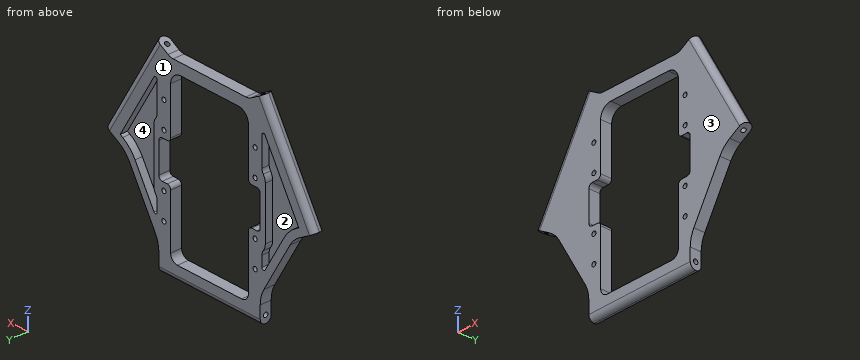
```python
from build123d import *

# Parameters (mm, degrees)
BOSS_EXTRUDE1_DEPTH = 6
SKETCH6_R           = 1.2
CUT_EXTRUDE1_DEPTH  = 104
SKETCH4_R           = 1.2
CUT_EXTRUDE2_DEPTH  = 104
SKETCH2_R           = 1.2
CUT_EXTRUDE3_DEPTH  = 104
FILLET2_R           = 3
SKETCH11_R          = 1.2
BOSS_EXTRUDE3_DEPTH = 32
SKETCH13_R          = 1.2
BOSS_EXTRUDE4_DEPTH = 32
BOSS_EXTRUDE5_START = -32
SKETCH14_R          = 1.2
BOSS_EXTRUDE5_DEPTH = 32
SKETCH16_W          = 46
SKETCH16_H          = 88
CUT_EXTRUDE5_DEPTH  = 10
SKETCH15_R          = 1.2
CUT_EXTRUDE4_DEPTH  = 10
FILLET3_R           = 6
FILLET1_R           = 16
FILLET4_R           = 6
FILLET5_R           = 4
CUT_EXTRUDE6_DEPTH  = 10
FILLET6_R           = 2
SKETCH18_R          = 1.2
CUT_EXTRUDE7_DEPTH  = 10
CUT_EXTRUDE8_DEPTH  = 4


with BuildPart() as part:
    # Sketch1 → Boss-Extrude1 (new body)
    with BuildSketch(Plane(origin=(0, 0, 0), x_dir=(1, 0, 0), z_dir=(0, 1, 0))):
        Polygon((-30, 54), (30, 54), (30, 40.038475773), (49.674337148, 5.961524227), (61.765371804, -1.019237886), (31.765371804, -52.980762114), (23.138438763, -48), (-23.138438763, -48), (-31.765371804, -52.980762114), (-61.765371804, -1.019237886), (-49.674337148, 5.961524227), (-30, 40.038475773), align=None)
    extrude(amount=BOSS_EXTRUDE1_DEPTH)

    # Sketch6 → Cut-Extrude1 (cut)
    with BuildSketch(Plane(origin=(15, 0, -25.980762114), x_dir=(-0.8660254037844389, 0, -0.4999999999999996), z_dir=(0.4999999999999996, 0, -0.8660254037844389))):
        with Locations((-50, 3)):
            Circle(SKETCH6_R)
    extrude(amount=-CUT_EXTRUDE1_DEPTH, mode=Mode.SUBTRACT)

    # Sketch4 → Cut-Extrude2 (cut)
    with BuildSketch(Plane(origin=(-15, 0, -25.980762114), x_dir=(-0.8660254037844386, 0, 0.5), z_dir=(-0.5000000000000001, 0, -0.8660254037844387))):
        with Locations((50, 3)):
            Circle(SKETCH4_R)
    extrude(amount=-CUT_EXTRUDE2_DEPTH, mode=Mode.SUBTRACT)

    # Sketch2 → Cut-Extrude3 (cut)
    with BuildSketch(Plane.ZY.offset(30)):
        with Locations((-50, 3)):
            Circle(SKETCH2_R)
    extrude(amount=-CUT_EXTRUDE3_DEPTH, mode=Mode.SUBTRACT)

    # Fillet2
    fillet2_edges = [part.edges().sort_by_distance(p)[0] for p in [
        (46.765371804, 0, 27),
        (46.765371804, 6, 27),
        (-46.765371804, 6, 27),
        (-46.765371804, 0, 27),
        (0, 0, -54),
        (0, 6, -54),
    ]]
    fillet(fillet2_edges, radius=FILLET2_R - 0.0001)  # a hair under: the kernel refuses the full size

    # Sketch11 → Boss-Extrude3 (add)
    with BuildSketch(Plane.ZY.offset(16)):
        with Locations((-50, 3)):
            Circle(SKETCH11_R)
    extrude(amount=-BOSS_EXTRUDE3_DEPTH)

    # Sketch13 → Boss-Extrude4 (add)
    with BuildSketch(Plane(origin=(8, 0, -13.856406461), x_dir=(-0.8660254037844386, 0, -0.4999999999999999), z_dir=(0.49999999999999994, 0, -0.8660254037844387))):
        with Locations((-50, 3)):
            Circle(SKETCH13_R)
    extrude(amount=-BOSS_EXTRUDE4_DEPTH)

    # Sketch14 → Boss-Extrude5 (add)
    with BuildSketch(Plane(origin=(8, 0, 13.856406461), x_dir=(0.8660254037844386, 0, -0.4999999999999999), z_dir=(0.49999999999999994, 0, 0.8660254037844387)).offset(BOSS_EXTRUDE5_START)):
        with Locations(Location((-50, 3, 0), (0, 0, 180))):
            Circle(SKETCH14_R)
    extrude(amount=BOSS_EXTRUDE5_DEPTH)

    # Sketch16 → Cut-Extrude5 (cut)
    with BuildSketch(Plane(origin=(0, 6, 0), x_dir=(1, 0, 0), z_dir=(0, 1, 0))):
        with Locations((0, 2)):
            Rectangle(SKETCH16_W, SKETCH16_H)
    extrude(amount=-CUT_EXTRUDE5_DEPTH, mode=Mode.SUBTRACT)

    # Sketch15 → Cut-Extrude4 (cut)
    with BuildSketch(Plane(origin=(0, 6, 0), x_dir=(1, 0, 0), z_dir=(0, 1, 0))):
        with Locations(Location((27, 29, 0), (0, 0, 270))):
            Circle(SKETCH15_R)
        with Locations(Location((-27, 15, 0), (0, 0, 270))):
            Circle(SKETCH15_R)
        with Locations(Location((-27, 29, 0), (0, 0, 270))):
            Circle(SKETCH15_R)
        with Locations(Location((27, 15, 0), (0, 0, 270))):
            Circle(SKETCH15_R)
    extrude(amount=-CUT_EXTRUDE4_DEPTH, mode=Mode.SUBTRACT)

    # Fillet3
    fillet3_edges = [part.edges().sort_by_distance(p)[0] for p in [
        (-23, 3, 42),
        (23, 3, 42),
    ]]
    fillet(fillet3_edges, radius=FILLET3_R)

    # Fillet1
    fillet1_edges = [part.edges().sort_by_distance(p)[0] for p in [
        (30, 3, -40.038475773),
        (49.674337148, 3, -5.961524227),
        (-49.674337148, 3, -5.961524227),
        (-30, 3, -40.038475773),
    ]]
    fillet(fillet1_edges, radius=FILLET1_R)

    # Fillet4
    fillet4_edges = [part.edges().sort_by_distance(p)[0] for p in [
        (23.138438763, 3, 48),
        (-23.138438763, 3, 48),
    ]]
    fillet(fillet4_edges, radius=FILLET4_R)

    # Fillet5
    fillet5_edges = [part.edges().sort_by_distance(p)[0] for p in [
        (-23, 3, -46),
        (23, 3, -46),
    ]]
    fillet(fillet5_edges, radius=FILLET5_R)

    # Sketch17 → Cut-Extrude6 (cut)
    with BuildSketch(Plane(origin=(0, 6, 0), x_dir=(1, 0, 0), z_dir=(0, 1, 0))):
        with BuildLine():
            Line((23, 11), (28, 11))
            ThreePointArc((28, 11), (29.414213562, 10.414213562), (30, 9))
            Line((30, 9), (30, -7))
            ThreePointArc((30, -7), (29.414213562, -8.414213562), (28, -9))
            Line((28, -9), (23, -9))
            Line((23, -9), (23, 11))
        make_face()
        with BuildLine():
            Line((-30, 9), (-30, -7))
            ThreePointArc((-30, -7), (-29.414213562, -8.414213562), (-28, -9))
            Line((-28, -9), (-23, -9))
            Line((-23, -9), (-23, 11))
            Line((-23, 11), (-28, 11))
            ThreePointArc((-28, 11), (-29.414213562, 10.414213562), (-30, 9))
        make_face()
    extrude(amount=-CUT_EXTRUDE6_DEPTH, mode=Mode.SUBTRACT)

    # Fillet6
    fillet6_edges = [part.edges().sort_by_distance(p)[0] for p in [
        (23, 3, 9),
        (23, 3, -11),
        (-23, 3, -11),
        (-23, 3, 9),
    ]]
    fillet(fillet6_edges, radius=FILLET6_R)

    # Sketch18 → Cut-Extrude7 (cut)
    with BuildSketch(Plane(origin=(0, 6, 0), x_dir=(1, 0, 0), z_dir=(0, 1, 0))):
        with Locations(Location((27, -13, 0), (0, 0, 270))):
            Circle(SKETCH18_R)
        with Locations(Location((27, -27, 0), (0, 0, 270))):
            Circle(SKETCH18_R)
        with Locations(Location((-27, -13, 0), (0, 0, 270))):
            Circle(SKETCH18_R)
        with Locations(Location((-27, -27, 0), (0, 0, 270))):
            Circle(SKETCH18_R)
    extrude(amount=-CUT_EXTRUDE7_DEPTH, mode=Mode.SUBTRACT)

    # Sketch19 → Cut-Extrude8 (cut)
    with BuildSketch(Plane(origin=(0, 6, 0), x_dir=(1, 0, 0), z_dir=(0, 1, 0))):
        with BuildLine():
            Line((31, 26.574374158), (31, 21))
            ThreePointArc((31, 21), (31.205266808, 19.735088936), (31.8, 18.6))
            ThreePointArc((31.8, 18.6), (32.692099788, 16.897366596), (33, 15))
            Line((33, 15), (33, -13))
            ThreePointArc((33, -13), (32.692099788, -14.897366596), (31.8, -16.6))
            ThreePointArc((31.8, -16.6), (31.205266808, -17.735088936), (31, -19))
            Line((31, -19), (31, -34.574374158))
            ThreePointArc((31, -34.574374158), (31.741180955, -35.540299984), (32.866025404, -35.074374158))
            Line((32.866025404, -35.074374158), (52.837168574, -0.483339502))
            Line((52.837168574, -0.483339502), (51.387150069, 0.353829072))
            ThreePointArc((51.387150069, 0.353829072), (47.245014446, 3.532201524), (44.066641994, 7.674337148))
            Line((44.066641994, 7.674337148), (32.866025404, 27.074374158))
            ThreePointArc((32.866025404, 27.074374158), (31.741180955, 27.540299984), (31, 26.574374158))
        make_face()
        with BuildLine():
            Line((-52.837168574, -0.483339502), (-32.866025404, -35.074374158))
            ThreePointArc((-32.866025404, -35.074374158), (-31.741180955, -35.540299984), (-31, -34.574374158))
            Line((-31, -34.574374158), (-31, -19))
            ThreePointArc((-31, -19), (-31.205266808, -17.735088936), (-31.8, -16.6))
            ThreePointArc((-31.8, -16.6), (-32.692099788, -14.897366596), (-33, -13))
            Line((-33, -13), (-33, 15))
            ThreePointArc((-33, 15), (-32.692099788, 16.897366596), (-31.8, 18.6))
            ThreePointArc((-31.8, 18.6), (-31.205266808, 19.735088936), (-31, 21))
            Line((-31, 21), (-31, 26.574374158))
            ThreePointArc((-31, 26.574374158), (-31.741180955, 27.540299984), (-32.866025404, 27.074374158))
            Line((-32.866025404, 27.074374158), (-44.066641994, 7.674337148))
            ThreePointArc((-44.066641994, 7.674337148), (-47.245014446, 3.532201524), (-51.387150069, 0.353829072))
            Line((-51.387150069, 0.353829072), (-52.837168574, -0.483339502))
        make_face()
    extrude(amount=-CUT_EXTRUDE8_DEPTH, mode=Mode.SUBTRACT)


solid = part.part
```
Read the model definition and answer for the solid it produces. Units are mm, in the model's axes. Face numbers are marked on the shaded views. A direction names the side the tool comes from. Give positions to 0.01 mm unless a question says otherwise; leave off trailing zeros. Answer as a JSON object with one key per item and string values.
1) For a pull along Z with two mould halves and no side action, classify the marked faces 3 and 4 as pulls with the +Z half, pulls with the -Z half, needs draft (parallel to the pull), parting line crosses it, or undercut.
Findings below:
{"face 3": "needs draft", "face 4": "undercut"}
2) A tool of negligible diameter and unlimited length cuts with its end or side. For the marked faces 1 and 2, from which of +Z, -Z, +X, -X, +Y, -Y can it reach the whole face along a straight path? Write none if from no direction.
Findings below:
{"face 1": "+Z, -Z, +X, -X, +Y", "face 2": "+Y"}
3) Flat-ended cylindrical pins translate along their axes: pin 1 Ø2 at (y, z) = (5, -27.5) entering from -X; pin 2 Ø3.5 at (x, y) = (-26, 3.5) entering from +Z; pin 3 Ø6.5 at (x, z) = (46, 4.5) entering from +Y; pin 4 Ø2 at (x, z) = (-27, 27) entering from +Y. Find the tip coordinate at first contact, or state that the pin passes through.
Findings below:
{"pin 1": "stops at x = -37.82", "pin 2": "stops at z = 50.63", "pin 3": "stops at y = 2", "pin 4": "passes through"}
4) Straight lines are drawn through the part: probe 1 along X at (y, z) = (1.55, -29); probe 2 along X at (y, z) = (1.95, -28); probe 3 along Y at (x, z) = (45, 12). For each, find the intervals that lie inside material, in ascending order. Write a range as from..to.
Findings below:
{"probe 1": "x = -36.37..-28.2, -25.8..-23, 23..25.8, 28.2..36.37", "probe 2": "x = -36.95..-27.66, -26.34..-23, 23..26.34, 27.66..36.95", "probe 3": "y = 0..2"}
